The listing builds one solid part. Answer for the finished solid, in the listing's coordinates (mm). A direction names the side the tool comes from. Round coordinates to 2 decimals unless told otherwise and drop trailing zeros. Write each loop counter-clockwise with the first axis right and the second up, starting at its lowest first coordinate (ties: lowest second). Pieces come first, ordered by that corner, then holes. Notation, with made-up numbers: (-15.5, 88) - (25.5, 88) arc R12 cw to (25.5, 107) - close; hole circle Ø10 at (0, 41). An arc over 180 degrees is marked (long way). Answer in a Markdown table with one row per item.
from build123d import *

# Parameters (mm, degrees)
BOSS_EXTRUDE1_DEPTH   = 9.675
SKETCH2_W             = 58.05
SKETCH2_H             = 3
BOSS_EXTRUDE1_2_DEPTH = 9.675
BOSS_EXTRUDE1_3_DEPTH = 9.675
BOSS_EXTRUDE2_DEPTH   = 3
BOSS_EXTRUDE3_DEPTH   = 12.675
SKETCH6_R             = 2.1
CUT_EXTRUDE1_DEPTH    = 43.959945007
SKETCH7_R             = 5
CUT_EXTRUDE2_DEPTH    = 1.5
SKETCH8_R             = 4.2
CUT_EXTRUDE3_DEPTH    = 5.2
CHAMFER1_SIZE         = 1.1
SKETCH9_R             = 7.55
CUT_EXTRUDE4_DEPTH    = 2
REVOLVE1_ANGLE        = 180


with BuildPart() as part:
    # Sketch2 → Boss-Extrude1 (new body)
    with BuildSketch(Plane(origin=(0, 0, 0), x_dir=(0, 0, -1), z_dir=(1, 0, 0))):
        Polygon((-29.025, 9.675), (-29.025, 12.675), (-12.675, 29.025), (-9.675, 29.025), (-9.675, 9.675), align=None)
    extrude(amount=-BOSS_EXTRUDE1_DEPTH)



with BuildPart() as body_2:
    # Sketch2 → Boss-Extrude1 2 (new body)
    with BuildSketch(Plane(origin=(0, 0, 0), x_dir=(0, 0, -1), z_dir=(1, 0, 0))):
        with Locations((0, -11.175)):
            Rectangle(SKETCH2_W, SKETCH2_H)
    extrude(amount=-BOSS_EXTRUDE1_2_DEPTH)


with BuildPart() as body_3:
    # Sketch2 → Boss-Extrude1 3 (new body)
    with BuildSketch(Plane(origin=(0, 0, 0), x_dir=(0, 0, -1), z_dir=(1, 0, 0))):
        Polygon((9.675, 29.025), (12.675, 29.025), (29.025, 12.675), (29.025, 9.675), (9.675, 9.675), align=None)
    extrude(amount=-BOSS_EXTRUDE1_3_DEPTH)


with BuildPart() as part_1:
    add(part.part)

    add(body_2.part)  # Boss-Extrude2 merges body 2

    add(body_3.part)  # Boss-Extrude2 merges body 3
    # Sketch3 → Boss-Extrude2 (add)
    with BuildSketch(Plane.ZY.offset(9.675)):
        Polygon((-29.025, 12.675), (-12.675, 29.025), (12.675, 29.025), (29.025, 12.675), (29.025, -12.675), (-29.025, -12.675), align=None)
    extrude(amount=BOSS_EXTRUDE2_DEPTH)

    # Sketch5 → Boss-Extrude3 (add)
    with BuildSketch(Plane(origin=(0, 0, 0), x_dir=(0, 0, -1), z_dir=(1, 0, 0))):
        with BuildLine():
            Line((-29.025, -12.675), (-23.675, -12.675))
            ThreePointArc((-23.675, -12.675), (-20.846572875, -13.846572875), (-19.675, -16.675))
            ThreePointArc((-19.675, -16.675), (-12.675, -23.675), (-5.675, -16.675))
            ThreePointArc((-5.675, -16.675), (-4.503427125, -13.846572875), (-1.675, -12.675))
            Line((-1.675, -12.675), (1.675, -12.675))
            ThreePointArc((1.675, -12.675), (4.503427125, -13.846572875), (5.675, -16.675))
            ThreePointArc((5.675, -16.675), (12.675, -23.675), (19.675, -16.675))
            ThreePointArc((19.675, -16.675), (20.846572875, -13.846572875), (23.675, -12.675))
            Line((23.675, -12.675), (29.025, -12.675))
            Line((29.025, -12.675), (29.025, -9.675))
            Line((29.025, -9.675), (-29.025, -9.675))
            Line((-29.025, -9.675), (-29.025, -12.675))
        make_face()
    extrude(amount=-BOSS_EXTRUDE3_DEPTH)

    # Sketch6 → Cut-Extrude1 (cut, through all)
    with BuildSketch(Plane(origin=(0, 0, 0), x_dir=(0, 0, -1), z_dir=(1, 0, 0))):
        with Locations((-12.675, -16.675)):
            Circle(SKETCH6_R)
        with Locations((12.675, -16.675)):
            Circle(SKETCH6_R)
        with Locations((-16.22116344, 16.22116344)):
            Circle(SKETCH6_R)
        with Locations(Location((16.22116344, 16.22116344, 0), (0, 0, 180))):
            Circle(SKETCH6_R)
    extrude(amount=-CUT_EXTRUDE1_DEPTH, mode=Mode.SUBTRACT)

    # Sketch7 → Cut-Extrude2 (cut)
    with BuildSketch(Plane.ZY.offset(12.675)):
        with Locations((-16.22116344, 16.22116344)):
            Circle(SKETCH7_R)
        with Locations((16.22116344, 16.22116344)):
            Circle(SKETCH7_R)
        with Locations((-12.675, -16.675)):
            Circle(SKETCH7_R)
        with Locations((12.675, -16.675)):
            Circle(SKETCH7_R)
    extrude(amount=-CUT_EXTRUDE2_DEPTH, mode=Mode.SUBTRACT)

    # Sketch8 → Cut-Extrude3 (cut)
    with BuildSketch(Plane(origin=(0, 0, 0), x_dir=(0, 0, -1), z_dir=(1, 0, 0))):
        with Locations((-16.22116344, 16.22116344)):
            Circle(SKETCH8_R)
        with Locations((16.22116344, 16.22116344)):
            Circle(SKETCH8_R)
        with Locations((12.675, -16.675)):
            Circle(SKETCH8_R)
        with Locations((-12.675, -16.675)):
            Circle(SKETCH8_R)
    extrude(amount=-CUT_EXTRUDE3_DEPTH, mode=Mode.SUBTRACT)

    # Chamfer1
    chamfer1_edges = [part_1.edges().sort_by_distance(p)[0] for p in [
        (0, -16.675, 16.875),
        (0, -16.675, -8.475),
        (0, 16.22116344, -12.02116344),
        (0, 16.22116344, 20.42116344),
    ]]
    chamfer(chamfer1_edges, length=CHAMFER1_SIZE)

    # Sketch9 → Cut-Extrude4 (cut)
    with BuildSketch(Plane(origin=(0, -9.675, 0), x_dir=(1, 0, 0), z_dir=(0, 1, 0))):
        Circle(SKETCH9_R)
    extrude(amount=-CUT_EXTRUDE4_DEPTH, mode=Mode.SUBTRACT)

    # Sketch10 → Revolve1 (revolve)
    with BuildSketch(Plane(origin=(0, 0, 0), x_dir=(0, 0, -1), z_dir=(1, 0, 0))):
        with BuildLine():
            Line((0, -15.975), (0, -11.675))
            Line((0, -11.675), (-10.731723594, -11.675))
            ThreePointArc((-10.731723594, -11.675), (-5.780568556, -14.860004257), (0, -15.975))
        make_face()
    revolve(axis=Axis((0, -15.975, 0), (0, -1, 0)), revolution_arc=REVOLVE1_ANGLE)

    # Sketch11 → Cut-Revolve1 (revolve, cut)
    with BuildSketch(Plane(origin=(0, 0, 0), x_dir=(0, 0, -1), z_dir=(1, 0, 0))):
        with BuildLine():
            Line((0, -13.975), (0, -11.675))
            Line((0, -11.675), (-7.55, -11.675))
            ThreePointArc((-7.55, -11.675), (-3.946279894, -13.387244869), (0, -13.975))
        make_face()
    revolve(axis=Axis((0, -13.975, 0), (0, 1, 0)), mode=Mode.SUBTRACT)


solid = part_1.part
(1) For a pull along Z with two mould halves and no side action, classify faces 1 (the flat face through (-12.675, 3, 0)), 2 (the flat face through (-10, 0, -29.025)), 3 (the flat face through (-11, -12.675, 0)), 4 (the cylindrical face through (-8.15, 16.31, 18.32)) as pulls with the +Z half, pulls with the -Z half, needs draft (parallel to the pull), parting line crosses it, or undercut.
Checked values:
| item | result |
|---|---|
| face 1 | needs draft |
| face 2 | pulls with the -Z half |
| face 3 | undercut |
| face 4 | undercut |
(2) Find the intervals of material crossed by line 1 (Z direction, x = -9, y = 16) (3 decimals); line 2 (Y direction, x = -9, z = -13) (3 decimals); line 3 (X direction, y = 20, z = 8.5) (3 decimals), in increasing order.
Checked values:
| item | result |
|---|---|
| line 1 | z = -25.7 to -18.309, -14.133 to -9.675, 9.675 to 14.133, 18.309 to 25.7 |
| line 2 | y = -23.667 to -18.75, -14.6 to -9.675, 9.675 to 28.7 |
| line 3 | x = -12.675 to -9.675 |
(3) Section A-A (x = -3.5) is taken. State how many separate pieces and enclosed holes the cut face has, and give its area (3 significant figures).
Checked values:
| item | result |
|---|---|
| separate pieces | 3 |
| enclosed holes | 4 |
| area | 693 mm2 |
(4) Section D-D (x = -10.5) is taken. Give the vertices of the cut face in (y, z) (3 decimals), and give its area (3 significant figures).
Checked values:
| item | result |
|---|---|
| outline | (-16.675, -19.675) arc R4 cw to (-12.675, -23.675) - (-12.675, -29.025) - (12.675, -29.025) - (29.025, -12.675) - (29.025, 12.675) - (12.675, 29.025) - (-12.675, 29.025) - (-12.675, 23.675) arc R4 cw to (-16.675, 19.675) arc R7 ccw to (-16.675, 5.675) arc R4 cw to (-12.675, 1.675) - (-12.675, -1.675) arc R4 cw to (-16.675, -5.675) arc R7 ccw to start; hole circle Ø4.2 at (-16.675, -12.675); hole circle Ø4.2 at (-16.675, 12.675); hole circle Ø4.2 at (16.221, -16.221); hole circle Ø4.2 at (16.221, 16.221) |
| area | 2,380 mm2 |
(5) Section B-B (y = 23) is taken. Give the vertices of the cut face in (x, z) (3 decimals).
Checked values:
| item | result |
|---|---|
| outline | (-12.675, -18.7) - (0, -18.7) - (0, -9.675) - (-9.675, -9.675) - (-9.675, 9.675) - (0, 9.675) - (0, 18.7) - (-12.675, 18.7) - close |
(6) Flat-ended cylindrical pins translate along their axes: pin 1 (2.5 mm diameter, centred on x = -9, z = -27, fed in from -Y) (3 decimals); pin 2 (5 mm diameter, centred on y = -17, z = -10.5, fed in from -X) (3 decimals); pin 3 (2 mm diameter, centred on x = -9, z = 10.5, fed in from -Y). Find the tip coordinate at first contact, or state that the pin passes through.
Checked values:
| item | result |
|---|---|
| pin 1 | stops at y = -12.675 |
| pin 2 | stops at x = -11.175 |
| pin 3 | stops at y = -23.58 |
(7) Section C-C (z = 0) is taken. Give the vertices of the cut face in (x, y) (3 decimals).
Checked values:
| item | result |
|---|---|
| outline | (-12.675, -12.675) - (-9.575, -12.675) arc R15.542 ccw to (0, -15.975) - (0, -13.975) arc R13.542 cw to (-7.55, -11.675) - (-7.55, -9.675) - (-9.675, -9.675) - (-9.675, 29.025) - (-12.675, 29.025) - close |
(8) For faces 5 (the flat face through (-5, 9.675, -19)), 6 (the cylindrical face through (-11.936, 16.441, -21.216)), 7 (the cylindrical face through (-3.121, 19.06, 19.317)), 8 (the cylindrical face through (-7.657, -14.345, -4.926)), determine the directions among +Z, -Z, +X, -X, +Y, -Y from which every point of the face is accessible in a straight line to the end or side of a thin tool.
Checked values:
| item | result |
|---|---|
| face 5 | +Z, -Z, +X |
| face 6 | -X |
| face 7 | +X |
| face 8 | -X, -Y |
